from build123d import *

# Parameters (mm, degrees)
F2_R = 0.508


# Not quite as in the source:
# - a fillet or chamfer that OpenCascade refuses, or shapes differently, is made with other operations: its cross-section is extruded or revolved along the edge and cut away or added


with BuildPart() as f1:
    # F0 (on Front) → F1 (revolve)
    with BuildSketch(Plane.XZ):
        with BuildLine():
            Line((-19.05, 0), (0, 0))
            ThreePointArc((0, 0), (-0.8365584984, 2.1276164223), (-3.1208319045, 2.034467252))
            Line((-3.1208319045, 2.034467252), (-3.1208319045, 0.891467252))
            Line((-3.1208319045, 0.891467252), (-4.0098319045, 0.891467252))
            ThreePointArc((-4.0098319045, 0.891467252), (-8.6732915332, 4.1995590152), (-13.335, 0.889))
            Line((-13.335, 0.889), (-13.335, 3.81))
            Line((-13.335, 3.81), (-15.24, 3.81))
            Line((-15.24, 3.81), (-15.24, 10.16))
            Line((-15.24, 10.16), (-19.05, 10.16))
            Line((-19.05, 10.16), (-19.05, 0))
        make_face()
    revolve(axis=Axis((-9.525, 0, 0), (-1, 0, 0)))

    # F2
    f2_edges = [f1.edges().sort_by_distance(p)[0] for p in [
        (-4.009832, 0, -0.891467),
        (-13.335, 0, -0.889),
        (-8.673292, 0, 4.199559),
    ]]
    fillet(f2_edges, radius=F2_R)

    # F3: chamfer of 0.762 on 3 edges, made by hand

    # F3_s1 → F3_t2 (revolve, cut)
    with BuildSketch(Plane.XZ):
        Polygon((-15.24, 9.398), (-16.002, 10.16), (-15.24, 10.16), align=None)
    revolve(axis=Axis((-15.24, 0, 0), (-1, 0, 0)), mode=Mode.SUBTRACT)

    # F3_s3 → F3_t4 (revolve, cut)
    with BuildSketch(Plane.XZ):
        Polygon((-13.335, 3.048), (-14.097, 3.81), (-13.335, 3.81), align=None)
    revolve(axis=Axis((-13.335, 0, 0), (-1, 0, 0)), mode=Mode.SUBTRACT)

    # F3_s5 → F3_t6 (revolve, cut)
    with BuildSketch(Plane.XZ):
        with BuildLine():
            Line((-3.1208319045, 1.600505207), (-2.6395418811, 2.3089160405))
            ThreePointArc((-2.6395418811, 2.3089160405), (-2.8778866419, 2.1954632748), (-3.1208319045, 2.034467252))
            Line((-3.1208319045, 2.034467252), (-3.1208319045, 1.600505207))
        make_face()
    revolve(axis=Axis((-3.1208319045, 0, 0), (-1, 0, 0)), mode=Mode.SUBTRACT)


solid = f1.part
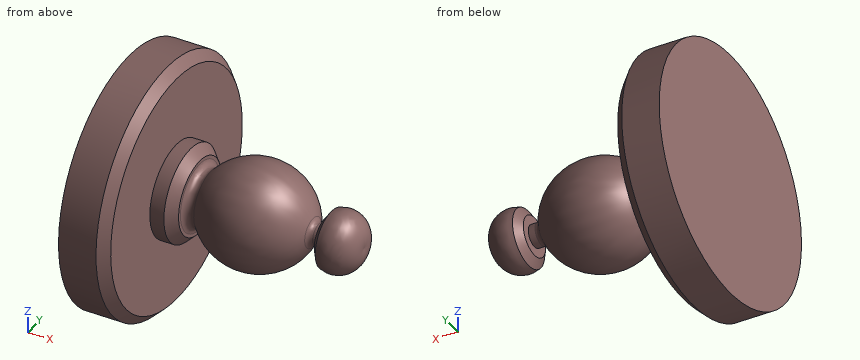
Design review of the part built by this model. Coordinates are the model's own, in mm. Coordinates: 2 decimals unless noted, no trailing zeros. Loops run counter-clockwise (first coordinate to the right, second up) from the corner with the lowest first, then second, coordinate; pieces in that order, holes last. Notation, with made-up numbers: (29, 22) -> (62, 22) arc R22 cw to (62, 37) -> close; hole circle Ø2 at (69, 55). An arc over 180 degrees is marked (long way). Use a Markdown table: item, result. Add a question column.
Item 1: Wall thickness on L1, parallel to X at y = -4.75, z = 4.25; L2, parallel to X at y = 3, z = 0 (3 decimals); L3, parallel to X at y = 2.5, z = -2.75: over which ranges is each line inside the solid? List them lowest first. Write a range as from..to.
Item 2: We need section A-A, the plane x = -16.75. Write out the cut boundary in (y, z), and give its area (3 significant figures).
Item 3: Clearance check with flat-ended pins moving along their axes: P1, Ø4, axis at x = -10, z = -7, coming from the +Y side; P2, Ø8, axis at x = -11, z = -7, coming from the +Y side; P3, Ø6, axis at y = 6.5, z = 6.5, coming from the +X side; P4, Ø6, axis at x = -8.5, z = -5.5, coming from the +Y side. State where each tip first meets the part, or that it passes through.
Numbers:
| question | item | result |
|---|---|---|
| 1 | L1 | x = -19.05..-15.24 |
| 1 | L2 | x = -19.05..-13.335, -11.899..-5.445 |
| 1 | L3 | x = -19.05..-14, -10.8..-6.54 |
| 2 | outline | circle Ø20.32 at (0, 0) |
| 2 | area | 324 mm^2 |
| 3 | P1 | passes through |
| 3 | P2 | stops at y = 2.53 |
| 3 | P3 | stops at x = -15.24 |
| 3 | P4 | stops at y = 3.37 |
